Model file for the job. Use its own axes, mm. Round coordinates to 2 decimals unless told otherwise and drop trailing zeros. Write each loop counter-clockwise with the first axis right and the second up, starting at its lowest first coordinate (ties: lowest second). Pieces come first, ordered by that corner, then holes. Notation, with made-up numbers: (3, 51) - (26, 51) arc R18 cw to (26, 85) - close; hole circle Ø4 at (42, 85.25). An arc over 180 degrees is marked (long way). One line per item, written item: value.
Autodesk Inventor part; units mm, degrees
ref_plane "YZ Plane" through (0, 0, 0) normal (1, 0, 0) x (0, 1, 0)
ref_plane "XZ Plane" through (0, 0, 0) normal (0, 1, 0) x (-1, 0, 0)
ref_plane "XY Plane" through (0, 0, 0) normal (0, 0, 1) x (1, 0, 0)
sketch "Sketch1" plane through (0, 0, 0) normal (1, 0, 0) x (0, 1, 0)
  line L0 (0, 0) -> (57.15, 0)
  line L1 (57.15, 0) -> (57.15, 20.32)
  line L2 (0, 0) -> (0, 20.32)
  line L3 (28.575, 0) -> (28.575, 8.5438) construction
  circle A0 centre (3.81, 3.81) radius 1.4
  circle A1 centre (53.34, 3.81) radius 1.4
  circle A2 centre (53.34, 16.51) radius 1.4
  circle A3 centre (3.81, 16.51) radius 1.4
  line L4 (0, 20.32) -> (57.15, 20.32)
  dimension "d0" = 57.15
  dimension "d1" = 20.32
  dimension "d2" = 20.32
  dimension "d5" = 2.8
  dimension "d6" = 3.81
  dimension "d7" = 3.81
  dimension "d14" = 2.8
  dimension "d15" = 12.7
  dimension "d18" = 49.53
extrude "Extrusion1" add sketch "Sketch1" along normal blind 1.6
properties part number "PCBModuleLeft02" material "PCB(1)"
1. Wall check: probe 1 along Z at (x, y) = (0.7, 3.81); probe 2 along Y at (x, z) = (1.1, 3.5); probe 3 along Z at (x, y) = (1.1, 5). Give the ranges that are in metal, low to high. Write a range as [from, to].
Report:
probe 1: [0, 2.41], [5.21, 15.11], [17.91, 20.32]
probe 2: [0, 2.44], [5.18, 51.97], [54.71, 57.15]
probe 3: [0, 3.07], [4.55, 15.77], [17.25, 20.32]
2. Mould opens along Y. For faces 1 (the face through (0, 28, 10)), 2 (the face through (0.79, 51.94, 3.75)), 3 (the face through (1, 0, 10)) say: released by +Y, released by -Y, zero draft, split by the parting line, or undercut.
Report:
face 1: zero draft
face 2: undercut
face 3: released by -Y
3. Band-saw the part on C-C on x = 0.9. Write the cut outline in (y, z).
Report:
outline: (0, 0) - (57.15, 0) - (57.15, 20.32) - (0, 20.32) - close; hole circle Ø2.8 at (3.81, 3.81); hole circle Ø2.8 at (3.81, 16.51); hole circle Ø2.8 at (53.34, 3.81); hole circle Ø2.8 at (53.34, 16.51)
4. Drop a flat-ended pin along its axis: pin 1 (10 mm diameter, centred on y = 24, z = 11, fed in from -X). Give the stop position or say it passes through.
Report:
pin 1: x = 0
5. Band-saw the part on A-A on y = 3.81. Write the cut outline in (x, z).
Report:
outline: (0, 0) - (1.6, 0) - (1.6, 2.41) - (0, 2.41) - close; (0, 5.21) - (1.6, 5.21) - (1.6, 15.11) - (0, 15.11) - close; (0, 17.91) - (1.6, 17.91) - (1.6, 20.32) - (0, 20.32) - close
6. Band-saw the part on B-B on z = 3.81. Write the cut outline in (x, y), plus the area to 3 significant figures.
Report:
outline: (0, 0) - (1.6, 0) - (1.6, 2.41) - (0, 2.41) - close; (0, 5.21) - (1.6, 5.21) - (1.6, 51.94) - (0, 51.94) - close; (0, 54.74) - (1.6, 54.74) - (1.6, 57.15) - (0, 57.15) - close
area: 82.5 mm²
